from build123d import *

# Parameters (mm, degrees)
F0_W      = 83.264
F0_H      = 127
F1_DEPTH  = 6.35
F2_W      = 15
F2_H      = 19.05
F3_DEPTH  = 26.67
F5_D      = 12.954
F7_D      = 6.528
F8_W      = 16
F8_H      = 20.828
F9_DEPTH  = 19.05
F11_DEPTH = 10
F13_DEPTH = 10
F15_D     = 9
F16_W     = 33.264
F16_H     = 28
F17_DEPTH = 6.351


# Not quite as in the source:
# - a feature names something its author has since deleted; it is built from what else it names


with BuildPart() as f1:
    # F0 (on Top) → F1 (new body)
    with BuildSketch(Plane.XY):
        with Locations((-3.6434741511, 1.1941809207)):
            Rectangle(F0_W, F0_H)
    extrude(amount=F1_DEPTH)

    # F2 (on face) → F3 (join)
    with BuildSketch(Plane.XY.offset(6.35)):
        with Locations((-37.7754741511, 55.1691809207)):
            Rectangle(F2_W, F2_H)
        with Locations((30.4885258489, 55.1691809207)):
            Rectangle(F2_W, F2_H)
        with Locations((30.4885258489, -52.7808190793)):
            Rectangle(F2_W, F2_H)
        with Locations((-37.7754741511, -52.7808190793)):
            Rectangle(F2_W, F2_H)
    extrude(amount=F3_DEPTH)

    # F5 (through all)
    with Locations(Plane(origin=(-45.2754741511, 0, 0), x_dir=(0, -1, 0), z_dir=(-1, 0, 0))):
        with Locations((-55.1691809207, 24.006), (52.7808190793, 24.006)):
            Hole(F5_D / 2)

    # F7 (through all)
    with Locations(Plane.XY.offset(6.35)):
        with Locations((-22.3994741511, 55.0421809207), (15.1125258489, 55.0421809207), (-22.3994741511, -52.6538190793), (15.1125258489, -52.6538190793)):
            Hole(F7_D / 2)

    # F8 (on face) → F9 (join)
    with BuildSketch(Plane.XY.offset(6.35)):
        with Locations((-31.2754741511, 1.1941809207)):
            Rectangle(F8_W, F8_H)
        with Locations((23.9885258489, 1.1941809207)):
            Rectangle(F8_W, F8_H)
    extrude(amount=F9_DEPTH)

    # F10 (on face) → F11 (cut)
    with BuildSketch(Plane(origin=(-39.2754741511, 0, 0), x_dir=(0, -1, 0), z_dir=(-1, 0, 0))):
        Polygon((5.1458190793, 13.4845992933), (5.1458190793, 20.8054007067), (-1.1941809207, 24.4658014133), (-7.5341809207, 20.8054007067), (-7.5341809207, 13.4845992933), (-1.1941809207, 9.8241985867), align=None)
    extrude(amount=-F11_DEPTH, mode=Mode.SUBTRACT)

    # F12 (on face) → F13 (cut)
    with BuildSketch(Plane.YZ.offset(31.9885258489)):
        Polygon((7.5341809207, 13.4845992933), (7.5341809207, 20.8054007067), (1.1941809207, 24.4658014133), (-5.1458190793, 20.8054007067), (-5.1458190793, 13.4845992933), (1.1941809207, 9.8241985867), align=None)
    extrude(amount=-F13_DEPTH, mode=Mode.SUBTRACT)

    # F15 (through all)
    with Locations(Plane(origin=(-29.2754741511, 0, 0), x_dir=(0, -1, 0), z_dir=(-1, 0, 0))):
        with Locations((-1.1941809207, 17.1448014133)):
            Hole(F15_D / 2)

    # F16 (on face) → F17 (cut, through all)
    with BuildSketch(Plane.XY.offset(6.35)):
        with Locations((-3.6434741511, 29.6941809207)):
            Rectangle(F16_W, F16_H)
        with Locations((-3.6434741511, -27.3058190793)):
            Rectangle(F16_W, F16_H)
    extrude(amount=-F17_DEPTH, mode=Mode.SUBTRACT)


solid = f1.part
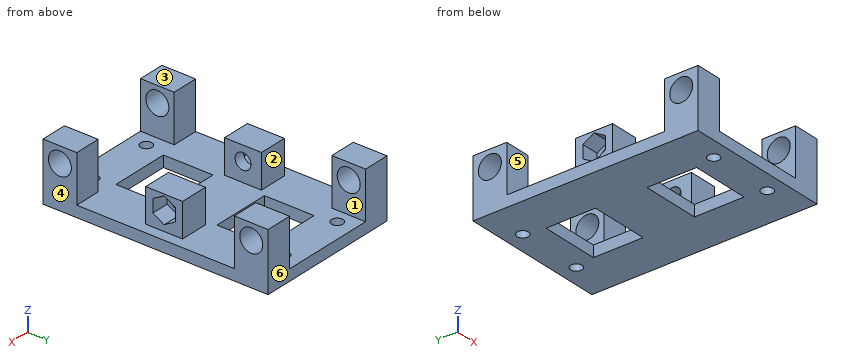
Check sheet for the modelled part. Datum: model origin and axes. Units: mm. Face numbers are marked on the shaded views. A direction names the side the tool comes from. Give positions to 0.01 mm unless a question says otherwise; leave off trailing zeros. Write each loop counter-clockwise with the first axis right and the second up, starting at its lowest first coordinate (ties: lowest second). Pieces come first, ordered by that corner, then holes. Notation, with made-up numbers: (57, 15.25) -> (82, 15.25) arc R9 cw to (82, 19.25) -> close; hole circle Ø7 at (-19.5, 21.5). An arc over 180 degrees is marked (long way). One line per item, written item: value. Start each with the question number.
Item 1: Section check C-C on y = -29. Record the cut outline in (x, z).
Item 2: Gauge pin test, flat ends, axial feed: pin 1 (7.5 mm diameter, centred on x = -22.4, y = 55.04, fed in from +Z); pin 2 (11.5 mm diameter, centred on y = 1.19, z = 17.14, fed in from -X); pin 3 (1.5 mm diameter, centred on x = 23.5, y = 11, fed in from +Z). Record the tip position at first contact, or that the pin passes through.
Item 3: Material ranges on probe 1 along Y at (x, z) = (-31.5, 27); probe 2 along X at (y, z) = (-8, 16.5); probe 3 along Y at (x, z) = (-29.5, 20), recorded low to high. Write a range as from..to.
Item 4: Section check A-A on z = 8. Record the cut outline in (x, y), then the cut area to 3 significant figures.
Item 5: Section check B-B on x = -15.5. Record the cut outline in (y, z).
Item 6: Draft check along Y on the marked faces 4, 5 and 6. Enter one of: +Y half, -Y half, draft (parallel to the pull), parting line (faces both ways), or undercut.
Item 7: Tool access check on the marked faces 1, 2 and 3. Record the directions out of +Z, -Z, +X, -X, +Y, -Y that give a thin tool (end or side, any length) a straight path to the whole face; none if there is none.
Item 8: Section check D-D on y = -1.5. Record the cut outline in (x, z), then the cut area to 3 significant figures.
Results list:
1. outline: (-45.28, 0) -> (-20.28, 0) -> (-20.28, 6.35) -> (-45.28, 6.35) -> close; (12.99, 0) -> (37.99, 0) -> (37.99, 6.35) -> (12.99, 6.35) -> close
2. pin 1: z = 6.35
2. pin 2: x = -29.28
2. pin 3: z = 25.4
3. probe 1: -62.31..-58.52, -47.04..-43.26, 45.64..49.43, 60.91..64.69
3. probe 2: -39.28..-23.28, 15.99..31.99
3. probe 3: -9.22..-5.15, 7.53..11.61
4. outline: (-45.28, -62.31) -> (-30.28, -62.31) -> (-30.28, -43.26) -> (-45.28, -43.26) -> close; (-45.28, 45.64) -> (-30.28, 45.64) -> (-30.28, 64.69) -> (-45.28, 64.69) -> close; (-39.28, -9.22) -> (-23.28, -9.22) -> (-23.28, 11.61) -> (-39.28, 11.61) -> close; (15.99, -9.22) -> (31.99, -9.22) -> (31.99, 11.61) -> (15.99, 11.61) -> close; (22.99, -62.31) -> (37.99, -62.31) -> (37.99, -43.26) -> (22.99, -43.26) -> close; (22.99, 45.64) -> (37.99, 45.64) -> (37.99, 64.69) -> (22.99, 64.69) -> close
4. area: 1,810 mm²
5. outline: (-62.31, 0) -> (-41.31, 0) -> (-41.31, 6.35) -> (-62.31, 6.35) -> close; (-13.31, 0) -> (15.69, 0) -> (15.69, 6.35) -> (-13.31, 6.35) -> close; (43.69, 0) -> (64.69, 0) -> (64.69, 6.35) -> (43.69, 6.35) -> close
6. face 4: draft
6. face 5: undercut
6. face 6: +Y half
7. face 1: +Z, +Y
7. face 2: +Z, +X, -X
7. face 3: +Z, +X, -X, +Y, -Y
8. outline: (-45.28, 0) -> (37.99, 0) -> (37.99, 6.35) -> (31.99, 6.35) -> (31.99, 11.38) -> (21.99, 11.38) -> (21.99, 13.54) -> (15.99, 13.54) -> (15.99, 6.35) -> (-23.28, 6.35) -> (-23.28, 13.54) -> (-29.28, 13.54) -> (-29.28, 11.38) -> (-39.28, 11.38) -> (-39.28, 6.35) -> (-45.28, 6.35) -> close; (-39.28, 22.91) -> (-29.28, 22.91) -> (-29.28, 20.75) -> (-23.28, 20.75) -> (-23.28, 25.4) -> (-39.28, 25.4) -> close; (15.99, 20.75) -> (21.99, 20.75) -> (21.99, 22.91) -> (31.99, 22.91) -> (31.99, 25.4) -> (15.99, 25.4) -> close
8. area: 821 mm²
